from build123d import *

# Parameters (mm, degrees)
SKETCH_1_R             = 2.5
EXTRUDE_1_DEPTH        = 30.5
SKETCH_2_R             = 5.5
EXTRUDE_2_DEPTH        = 27.5
SKETCH_3_R             = 2.5
EXTRUDE_3_DEPTH        = 12
SKETCH_4_W             = 2
SKETCH_4_H             = 1
EXTRUDE_4_DEPTH        = 5
HOLE_WIZARD_M4_1_D     = 3.3
HOLE_WIZARD_M4_1_DEPTH = 10.508579979
HOLE_WIZARD_M4_1_TIP   = 0.991420021


with BuildPart() as part:
    # 草图1 → 凸台-拉伸1 (new, symmetric)
    with BuildSketch(Plane(origin=(0, 0, 0), x_dir=(1, 0, 0), z_dir=(0, 1, 0))):
        with Locations(Location((0, 0, 0), (0, 0, 90))):
            Circle(SKETCH_1_R)
    extrude(amount=EXTRUDE_1_DEPTH, both=True)

    # 草图2 → 凸台-拉伸2 (add, symmetric)
    with BuildSketch(Plane(origin=(0, 0, 0), x_dir=(1, 0, 0), z_dir=(0, 1, 0))):
        with Locations(Location((0, 0, 0), (0, 0, 270))):
            Circle(SKETCH_2_R)
    extrude(amount=EXTRUDE_2_DEPTH, both=True)

    # 草图3 → 凸台-拉伸3 (add)
    with BuildSketch(Plane.XZ.offset(30.5)):
        with Locations(Location((0, 0, 0), (0, 0, 270))):
            Circle(SKETCH_3_R)
    extrude(amount=EXTRUDE_3_DEPTH)

    # 草图4 → 凸台-拉伸4 (add)
    with BuildSketch(Plane.XZ.offset(42.5)):
        with Locations((0, 2.5)):
            Rectangle(SKETCH_4_W, SKETCH_4_H)
    extrude(amount=-EXTRUDE_4_DEPTH)

    # M4 螺纹孔1
    with Locations(Plane(origin=(0, -42.5, 0), x_dir=(-1, 0, 0), z_dir=(0, -1, 0))):
        with Locations((0, 0)):
            Hole(HOLE_WIZARD_M4_1_D / 2, depth=HOLE_WIZARD_M4_1_DEPTH)
            with Locations((0, 0, -(HOLE_WIZARD_M4_1_DEPTH + HOLE_WIZARD_M4_1_TIP / 2))):  # 118° drill point
                Cone(0, HOLE_WIZARD_M4_1_D / 2, HOLE_WIZARD_M4_1_TIP, mode=Mode.SUBTRACT)


solid = part.part
Can you work these out from the model? Positions are in its coordinate system, mm. A direction names the side the tool comes from. Give positions to 0.01 mm unless a question says otherwise; leave off trailing zeros. Order: outer loops, then holes, each group sorted by start corner. A loop starts at its lowest first (then second) coordinate and runs counter-clockwise, first axis right, second up. Notation, with made-up numbers: M -21,28.25 L 18,28.25 A19 cw 18,55.25 Z; hole C 6,1.25 d11. An arc over 180 degrees is marked long. One line per item, written item: value.
Item 1: For faces 4 (the face through (-5.37, 0.39, -1.19)), 5 (the face through (2.44, 29.02, 0.54)), 6 (the face through (0, -40, 3)), which set-ups out of +Z, -Z, +X, -X, +Y, -Y let a thin tool reach every point of the face, with its end or its side?
Verdict:
face 4: +Y, -Y
face 5: +Y
face 6: +Z, +X, -X, -Y
Item 2: For pin 1 (1 mm diameter, centred on y = 4, z = 2, fed in from -X); pin 2 (2 mm diameter, centred on x = 0, y = -39.5, fed in from +Z); pin 3 (0.8 mm diameter, centred on x = -0.5, z = 3, fed in from +Y), each with a flat end and sliding along its axis, tell me the tip position at first contact or that it passes through.
Verdict:
pin 1: x = -5.29
pin 2: z = 3
pin 3: y = 27.5
Item 3: If we section it at A-A on y = -14.5: Write out the boundary of the cut face in (x, z).
Verdict:
outline: C 0,0 d11
Item 4: If we mould it in two halves opening along Z, with no side actions, what happens to faces 1 (the face through (0, -27.5, -3)), 2 (the face through (-1.216, -37.172, -1.115)), 3 (the face through (0.751, -34.895, -2.385))? For each: pulls with the +Z half, pulls with the -Z half, needs draft (parallel to the pull), parting line crosses it, or undercut.
Verdict:
face 1: needs draft
face 2: undercut
face 3: parting line crosses it
Item 5: Please list where these lines run through material, in increasing order: line 1 (Z direction, x = 0, y = -34.5); line 2 (Z direction, x = 0, y = -39); line 3 (Y direction, x = 0.75, z = 4.5).
Verdict:
line 1: -2.5 to -1.65, 1.65 to 2.5
line 2: -2.5 to -1.65, 1.65 to 3
line 3: -27.5 to 27.5
